Verification items for this drawing (mm, ordinates from the low corner). A direction names the side the tool comes from. Round coordinates to 2 decimals unless told otherwise and drop trailing zeros. Write each loop counter-clockwise with the first axis right and the second up, starting at its lowest first coordinate (ties: lowest second). Pieces come first, ordered by that corner, then holes.
Item 1: Depth check by flat-ended pin: P1, Ø2.5, axis at x = 35, z = 4.5, coming from the -Y side; P2, Ø4, axis at y = 30, z = 6, coming from the +X side; P3, Ø3.5, axis at y = 22.5, z = 6, coming from the +X side; P4, Ø2.5, axis at x = 84.5, z = 7, coming from the +Y side. Enter the tip coordinate at first touch or a pass-through.
Item 2: Access from +Z, -Z, +X, -X, +Y, -Y to the whole of each face (thin tool, end or side, straight path). Record for the marked faces 1 and 2.
Item 3: Cross-section at A-A (z = 10). Enter the section's corners in (x, y), then the cut area to 3 significant figures.
Item 4: Scan lines: probe 1 along X at (y, z) = (2.5, 0.95); probe 2 along Y at (x, z) = (2.5, 0.8); probe 3 along Z at (x, y) = (58.5, 28). Record each from-to range of solid material in increasing order.
Item 5: Cross-section at D-D (y = 11.5). Enter the section's corners in (x, z).
Item 6: Cross-section at B-B (x = 2.5). Enter the section's corners in (y, z).
Item 7: Cross-section at C-C (x = 72.5). Enter the section's corners in (y, z), then the cut area to 3 significant figures.
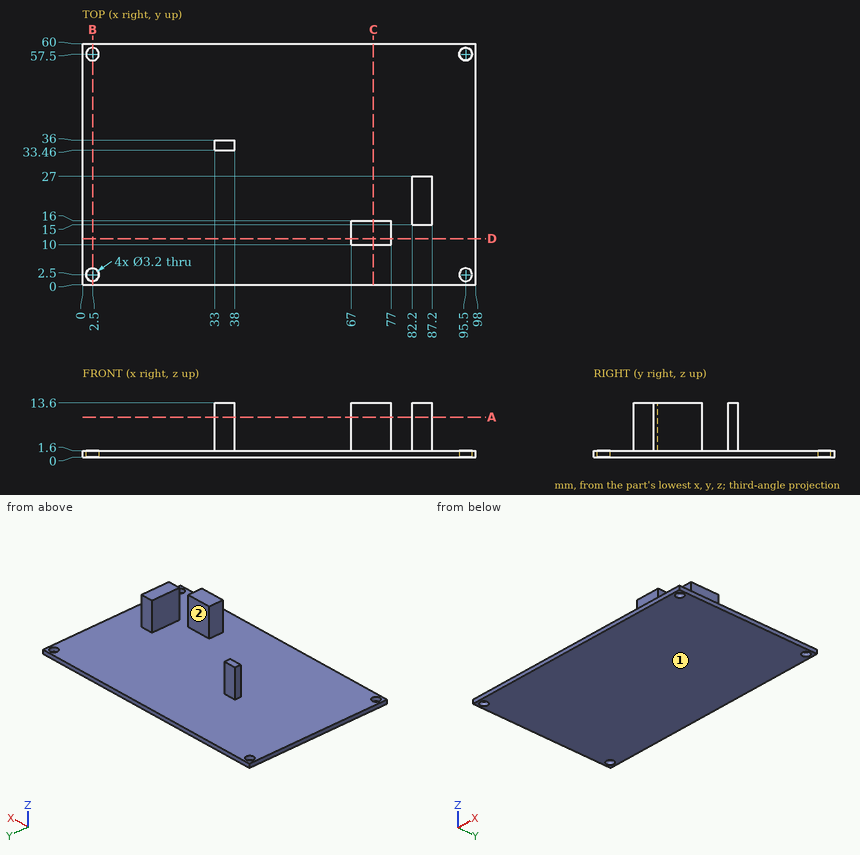
Resolved:
1. P1: stops at y = 33.46
1. P2: passes through
1. P3: stops at x = 87.2
1. P4: stops at y = 27
2. face 1: -Z, +X, -X, +Y, -Y
2. face 2: +Z, -X, +Y
3. outline: (33, 33.46) - (38, 33.46) - (38, 36) - (33, 36) - close; (67, 10) - (77, 10) - (77, 16) - (67, 16) - close; (82.2, 15) - (87.2, 15) - (87.2, 27) - (82.2, 27) - close
3. area: 133 mm2
4. probe 1: x = 0 to 0.9, 4.1 to 93.9, 97.1 to 98
4. probe 2: y = 0 to 0.9, 4.1 to 55.9, 59.1 to 60
4. probe 3: z = 0 to 1.6
5. outline: (0, 0) - (98, 0) - (98, 1.6) - (77, 1.6) - (77, 13.6) - (67, 13.6) - (67, 1.6) - (0, 1.6) - close
6. outline: (0, 0) - (0.9, 0) - (0.9, 1.6) - (0, 1.6) - close; (4.1, 0) - (55.9, 0) - (55.9, 1.6) - (4.1, 1.6) - close; (59.1, 0) - (60, 0) - (60, 1.6) - (59.1, 1.6) - close
7. outline: (0, 0) - (60, 0) - (60, 1.6) - (16, 1.6) - (16, 13.6) - (10, 13.6) - (10, 1.6) - (0, 1.6) - close
7. area: 168 mm2
